Verification items for the finished model (mm, model axes). A direction names the side the tool comes from. Round coordinates to 2 decimals unless told otherwise and drop trailing zeros. Write each loop counter-clockwise with the first axis right and the second up, starting at its lowest first coordinate (ties: lowest second). Pieces come first, ordered by that corner, then holes. Notation, with made-up numbers: M 45.25,81 L 87.25,81 A16 ccw 87.25,105 Z; hole C 76.25,-32.5 d1. An arc over 180 degrees is marked long. One line per question, with ' | ' between items. Start each with the question number.
Q1. Thickness scan on line 1 along Z through (x, y) = (0, 5.5); line 2 along Z through (x, y) = (0, 18.5); line 3 along Y through (x, z) = (3.75, 2.5). Record the ranges inside material, lowest first. Write a range as from..to.
Q2. Cross-section at C-C (z = -2.25). Record the boundary of the cut face in (x, y).
Q3. Tool access check on faces 1 (the face through (-1.3, 4, 5.7)), 2 (the face through (-3, 6, 0)). Record the directions out of +Z, -Z, +X, -X, +Y, -Y that give a thin tool (end or side, any length) a straight path to the whole face; none if there is none.
Q4. Release check for a two-part mould opening along Z. For faces 3 (the face through (-1.3, 4, -8.3)), 4 (the face through (5, 30, -3)) record: released by +Z, released by -Z, zero draft, split by the parting line, or undercut.
Q5. Gauge pin test, flat ends, axial feed: pin 1 (4 mm diameter, centred on x = 5.5, y = 24, fed in from -Z); pin 2 (1 mm diameter, centred on y = 25.5, z = -2.5, fed in from +X); pin 3 (3.5 mm diameter, centred on x = 0, z = 7, fed in from +Y); pin 4 (2.5 mm diameter, centred on x = 0, z = -7, fed in from +Y). Record the tip position at first contact, or that the pin passes through.
Q6. Cross-section at B-B (y = 25). Record the boundary of the cut face in (x, z).
Q7. Cross-section at D-D (y = 15.5). Record the boundary of the cut face in (x, z).
Autodesk Inventor part; units mm, degrees
ref_plane "YZ Plane" through (0, 0, 0) normal (1, 0, 0) x (0, 1, 0)
ref_plane "XZ Plane" through (0, 0, 0) normal (0, 1, 0) x (-1, 0, 0)
ref_plane "XY Plane" through (0, 0, 0) normal (0, 0, 1) x (1, 0, 0)
sketch "Boceto5" plane through (0, 0, 0) normal (0, 1, 0) x (-1, 0, 0)
  circle A0 centre (0, 0) radius 11
  line L0 (0, 0) -> (0, -7)
  line L1 (0, 0) -> (0, 7)
  circle A1 centre (0, 7) radius 1.5
  circle A2 centre (0, -7) radius 1.5
  dimension "d25" = 22
  dimension "d26" = 7
  dimension "d27" = 7
  dimension "d28" = 3
  dimension "d29" = 3
extrude "Extrusión6" add sketch "Boceto5" along normal blind 4
sketch "Boceto6" plane through (0, 4, 0) normal (0, 1, 0) x (1, 0, 0)
  circle A0 centre (0, 0) radius 11
  circle A1 centre (0, -7) radius 1.5
  circle A2 centre (0, -7) radius 3
  circle A3 centre (0, 7) radius 1.5
  circle A4 centre (0, 7) radius 3
  dimension "d32" = 6
  dimension "d33" = 6
extrude "Extrusión7" add sketch "Boceto6" along normal blind 8 contours A0
sketch "Boceto7" plane through (0, 12, 0) normal (0, 1, 0) x (1, 0, 0)
  circle A0 centre (0, 0) radius 5.25
  circle A1 centre (0, -7) radius 3
  circle A2 centre (0, -7) radius 3
  circle A3 centre (0, 7) radius 1.5
  circle A4 centre (0, 7) radius 3
  circle A5 centre (0, 0) radius 11
  dimension "d36" = 10.5
extrude "Extrusión8" add sketch "Boceto7" along normal blind 20 contours A5
sketch "Boceto8" plane through (0, 0, 0) normal (1, 0, 0) x (0, 1, 0)
  line L0 (0, 0) -> (23, 0)
  line L1 (23, 0) -> (25, 0)
  circle A0 centre (25, 0) radius 1.5
  dimension "d39" = 23
  dimension "d43" = 2
  dimension "d44" = 3
extrude "Extrusión10" cut sketch "Boceto8" along normal mid plane 22
move faces "Desplazar2" translate (0, -2, 0) faces at (5.0629, 32, -5.6904)
sketch "Boceto9" plane through (0, 0, 0) normal (0, -1, 0) x (1, 0, 0)
  circle A0 centre (0, 0) radius 3
  dimension "d52" = 6
extrude "Extrusión11" cut sketch "Boceto9" against normal blind 12
properties part number "end_effector_connector_arm2_grande"
Determined:
1) line 1: z = -11..-10, -4..-3, 3..4, 10..11 | line 2: z = -11..-10, 10..11 | line 3: y = 0..12
2) outline: M -10.77,0 L -1.98,0 L -1.98,12 L -4.74,12 L -4.74,30 L -10.77,30 Z; M 1.98,0 L 10.77,0 L 10.77,30 L 4.74,30 L 4.74,12 L 1.98,12 Z
3) face 1: +Y | face 2: +Y, -Y
4) face 3: undercut | face 4: zero draft
5) pin 1: stops at z = -10.43 | pin 2: stops at x = 10.82 | pin 3: stops at y = 4 | pin 4: passes through
6) outline: M -10.9,-1.5 A11 ccw 10.9,-1.5 L 5.03,-1.5 A5.25 cw 2.07,-4.83 A3 cw long -2.07,-4.83 A5.25 cw -5.03,-1.5 Z; M -10.9,1.5 L -5.03,1.5 A5.25 cw -2.07,4.83 A3 cw long 2.07,4.83 A5.25 cw 5.03,1.5 L 10.9,1.5 A11 ccw Z
7) outline: C 0,0 d22; hole M -2.07,-4.83 A3 ccw long 2.07,-4.83 A5.25 ccw 2.07,4.83 A3 ccw long -2.07,4.83 A5.25 ccw Z
